```python
from build123d import *

# Parameters (mm, degrees)
SKETCH1_R           = 21.971
BOSS_EXTRUDE1_DEPTH = 1.6256
SKETCH2_R           = 1.25
CUT_EXTRUDE1_DEPTH  = 32.114180969
SKETCH3_W           = 13.98846053
SKETCH3_H           = 5.196987607
CUT_EXTRUDE2_DEPTH  = 32.114180969


with BuildPart() as part:
    # Sketch1 → Boss-Extrude1 (new body)
    with BuildSketch(Plane.XY):
        Circle(SKETCH1_R)
    extrude(amount=BOSS_EXTRUDE1_DEPTH)

    # Sketch2 → Cut-Extrude1 (cut, through all)
    with BuildSketch(Plane.XY.offset(1.6256)):
        with Locations((12, 12)):
            Circle(SKETCH2_R)
        with Locations((-12, -12)):
            Circle(SKETCH2_R)
    extrude(amount=-CUT_EXTRUDE1_DEPTH, mode=Mode.SUBTRACT)

    # Sketch3 → Cut-Extrude2 (cut, through all)
    with BuildSketch(Plane(origin=(0, 0, 0), x_dir=(-1, 0, 0), z_dir=(0, 0, -1))):
        with Locations((0, 23.426493804)):
            Rectangle(SKETCH3_W, SKETCH3_H)
        with Locations((0, -23.426493804)):
            Rectangle(SKETCH3_W, SKETCH3_H)
    extrude(amount=-CUT_EXTRUDE2_DEPTH, mode=Mode.SUBTRACT)


solid = part.part
```
Check sheet for the modelled part. Datum: model origin and axes. Units: mm. Round coordinates to 2 decimals unless told otherwise and drop trailing zeros. Loops run counter-clockwise (first coordinate to the right, second up) from the corner with the lowest first, then second, coordinate; pieces in that order, holes last. Notation, with made-up numbers: (15.5, 60) - (35.5, 60) arc R21 cw to (35.5, 90) - close; hole circle Ø1 at (31.5, 28). An arc over 180 degrees is marked (long way). Answer as a JSON object with one key per item and string values. Group by question number.
Q1. Scan lines: line 1 along Y through (x, z) = (-12, 0.95); line 2 along X through (y, z) = (7, 0.6); line 3 along X through (y, z) = (-11.5, 0.2). Record each from-to range of solid material in increasing order. Write a range as [from, to].
Q2. Sectioned sample at A-A, the plane z = 0.6. Enter the section's corners in (x, y), plus the area to 3 significant figures.
Q3. Sectioned sample at C-C, the plane y = -12. Enter the section's corners in (x, z), plus the area to 3 significant figures.
Q4. Sectioned sample at D-D, the plane y = -4.5. Enter the section's corners in (x, z).
Q5. Sectioned sample at B-B, the plane x = 12. Enter the section's corners in (y, z).
Solution:
{
 "1": {"line 1": "y = [-18.4, -13.25], [-10.75, 18.4]", "line 2": "x = [-20.83, 20.83]", "line 3": "x = [-18.72, -13.15], [-10.85, 18.72]"},
 "2": {"outline": "(-6.99, -20.83) - (6.99, -20.83) arc R21.97 ccw to (6.99, 20.83) - (-6.99, 20.83) arc R21.97 ccw to start; hole circle Ø2.5 at (-12, -12); hole circle Ø2.5 at (12, 12)", "area": "1,490 mm²"},
 "3": {"outline": "(-18.4, 0) - (-13.25, 0) - (-13.25, 1.63) - (-18.4, 1.63) - close; (-10.75, 0) - (18.4, 0) - (18.4, 1.63) - (-10.75, 1.63) - close", "area": "55.8 mm²"},
 "4": {"outline": "(-21.51, 0) - (21.51, 0) - (21.51, 1.63) - (-21.51, 1.63) - close"},
 "5": {"outline": "(-18.4, 0) - (10.75, 0) - (10.75, 1.63) - (-18.4, 1.63) - close; (13.25, 0) - (18.4, 0) - (18.4, 1.63) - (13.25, 1.63) - close"}
}
